```python
from build123d import *

# Parameters (mm, degrees)
F0_W     = 99.75113
F0_H     = 86.922713
F1_DEPTH = 25.4
F2_T     = -1.27
F4_D     = 6.35
F6_D     = 6.35
F6_DEPTH = 12.7
F8_D     = 6.35
F8_DEPTH = 12.7


with BuildPart() as f1:
    # F0 (on Front) → F1 (new body)
    with BuildSketch(Plane.XZ):
        with Locations((49.875565, 43.461357)):
            Rectangle(F0_W, F0_H)
    extrude(amount=F1_DEPTH)

    # F2
    f2_openings = [f1.faces().sort_by_distance(p)[0] for p in [
        (49.875565, -25.4, 43.461356),
    ]]
    offset(amount=F2_T, openings=f2_openings)

    # F4 (through all)
    with Locations(Plane.YZ.offset(99.75113)):
        with Locations((-11.947631, 43.461356)):
            Hole(F4_D / 2)

    # F6
    with Locations(Plane.YZ.offset(1.27)):
        with Locations((-11.557093, 47.894768)):
            Hole(F6_D / 2, depth=F6_DEPTH)

    # F8
    with Locations(Plane.YZ.offset(99.75113)):
        with Locations((-12.7, 54.16663)):
            Hole(F8_D / 2, depth=F8_DEPTH)


solid = f1.part
```
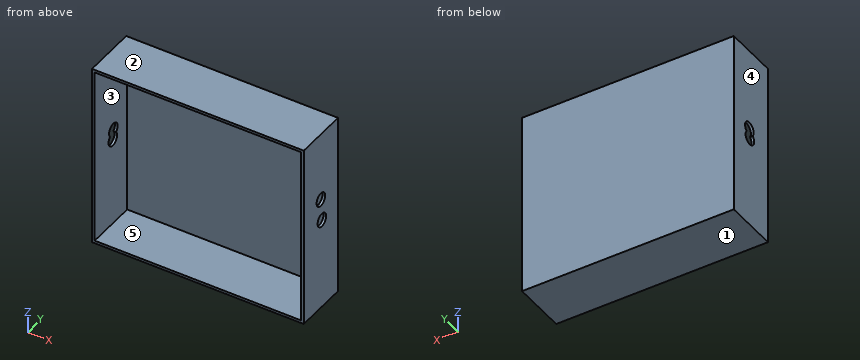
The model under review builds one solid part; all positions refer to its coordinate system, in mm. Face numbers are marked on the shaded views. A direction names the side the tool comes from. Round coordinates to 2 decimals unless told otherwise and drop trailing zeros. Loops run counter-clockwise (first coordinate to the right, second up) from the corner with the lowest first, then second, coordinate; pieces in that order, holes last. Notation, with made-up numbers: M -10,51 L -3,51 A32 ccw -3,79 Z; hole C 71,-29.75 d8. An arc over 180 degrees is marked long. Answer as a JSON object with one key per item and string values.
(1) Take a section at B-B on z = 80. Give the boundary of the cut face in (x, y), and give its area (3 significant figures).
Resolved:
{"outline": "M 0,-25.4 L 1.27,-25.4 L 1.27,-1.27 L 98.48,-1.27 L 98.48,-25.4 L 99.75,-25.4 L 99.75,0 L 0,0 Z", "area": "188 mm²"}
(2) To check wall thickness, follow line 1 along Z through (x, y) = (16, -14); line 2 along X through (y, z) = (-21, 47.5); line 3 along Z through (x, y) = (99.5, -12.7). State the ranges of each line that lie inside material, in increasing order.
Resolved:
{"line 1": "0 to 1.27, 85.65 to 86.92", "line 2": "0 to 1.27, 98.48 to 99.75", "line 3": "0 to 40.38, 46.55 to 50.99, 57.34 to 86.92"}
(3) Clearance check with flat-ended pins moving along their axes: P1, Ø10, axis at x = 71.5, z = 20.5, coming from the -Y side; P2, Ø2, axis at x = 76.5, z = 48.5, coming from the +Y side. State where each tip first meets the part, or that it passes through.
Resolved:
{"P1": "y = -1.27", "P2": "y = 0"}
(4) Take a section at D-D on y = -19.25. Give the boundary of the cut face in (x, z), and give its area (3 significant figures).
Resolved:
{"outline": "M 0,0 L 99.75,0 L 99.75,86.92 L 0,86.92 Z; hole M 1.27,1.27 L 98.48,1.27 L 98.48,85.65 L 1.27,85.65 Z", "area": "468 mm²"}
(5) Take a section at C-C on x = 78. Give the boundary of the cut face in (y, z), and give its area (3 significant figures).
Resolved:
{"outline": "M -25.4,0 L 0,0 L 0,86.92 L -25.4,86.92 L -25.4,85.65 L -1.27,85.65 L -1.27,1.27 L -25.4,1.27 Z", "area": "172 mm²"}
(6) Draft analysis for pull direction Z (two halves, no side actions). For the marked faces 1, 2 and 3, state which applies: released by +Z, released by -Z, zero draft, split by the parting line, or undercut.
Resolved:
{"face 1": "released by -Z", "face 2": "released by +Z", "face 3": "undercut"}
(7) Tool access review of the marked faces 4 and 5: name each direction out of +Z, -Z, +X, -X, +Y, -Y from which nothing blocks a thin tool from reaching the whole face with its end or side.
Resolved:
{"face 4": "+Z, -Z, -X, +Y, -Y", "face 5": "-Y"}
(8) Take a section at A-A on y = -12.7. Give the boundary of the cut face in (x, z), and give its area (3 significant figures).
Resolved:
{"outline": "M 0,0 L 99.75,0 L 99.75,40.38 L 98.48,40.38 L 98.48,1.27 L 1.27,1.27 L 1.27,40.38 L 0,40.38 Z; M 0,50.86 L 1.27,50.86 L 1.27,85.65 L 98.48,85.65 L 98.48,57.34 L 99.75,57.34 L 99.75,86.92 L 0,86.92 Z; M 98.48,46.55 L 99.75,46.55 L 99.75,50.99 L 98.48,50.99 Z", "area": "438 mm²"}
